Could you check a few things on this model? Use its own coordinates, in mm. Face numbers are marked on the shaded views. A direction names the side the tool comes from. Round coordinates to 2 decimals unless told otherwise and drop trailing zeros. Write each loop counter-clockwise with the first axis right and the second up, starting at its lowest first coordinate (ties: lowest second). Pieces come first, ordered by that corner, then holes. Notation, with made-up numbers: (36, 48.25) -> (56, 48.25) arc R22 ccw to (56, 71.25) -> close; hole circle Ø11 at (-4, 15.5). An arc over 180 degrees is marked (long way). Answer in a Markdown table with one row per item.
from build123d import *

# Parameters (mm, degrees)
BOSS_EXTRUDE1_DEPTH = 9


with BuildPart() as part:
    # Sketch1 → Boss-Extrude1 (new, symmetric)
    with BuildSketch(Plane.XY):
        with BuildLine():
            Line((10, 3.992849301), (10, -6.01853916))
            Line((10, -6.01853916), (5, -6.01853916))
            ThreePointArc((5, -6.01853916), (4.292893219, -6.311432379), (4, -7.01853916))
            Line((4, -7.01853916), (4, -8.007150699))
            Line((4, -8.007150699), (-4, -8.007150699))
            Line((-4, -8.007150699), (-4, -7.01853916))
            ThreePointArc((-4, -7.01853916), (-4.292893219, -6.311432379), (-5, -6.01853916))
            Line((-5, -6.01853916), (-10, -6.01853916))
            Line((-10, -6.01853916), (-10, 3.992849301))
            ThreePointArc((-10, 3.992849301), (0, 1.100511346), (10, 3.992849301))
        make_face()
    extrude(amount=BOSS_EXTRUDE1_DEPTH, both=True)


solid = part.part
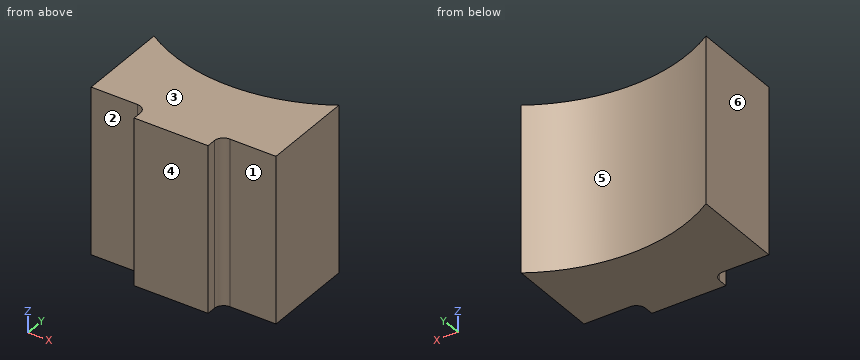
1) Imagine slicing it at A-A, the plane z = 1. Please give me the cut outline in (x, y).
Findings:
| item | result |
|---|---|
| outline | (-10, -6.02) -> (-5, -6.02) arc R1 cw to (-4, -7.02) -> (-4, -8.01) -> (4, -8.01) -> (4, -7.02) arc R1 cw to (5, -6.02) -> (10, -6.02) -> (10, 3.99) arc R18.73 cw to (-10, 3.99) -> close |
2) Thinking about a two-plate mould opening in X: for the marked faces 4, 5 and 6, which applies, +X half, -X half, draft (parallel to the pull), parting line (faces both ways), or undercut?
Findings:
| item | result |
|---|---|
| face 4 | draft |
| face 5 | undercut |
| face 6 | -X half |
3) Please list where these lines run through material, in increasing order: line 1 (X direction, y = 3, z = 2.25); line 2 (Y direction, x = 4.5, z = 2); line 3 (Y direction, x = -2.25, z = -7).
Findings:
| item | result |
|---|---|
| line 1 | x = -10 to -8.22, 8.22 to 10 |
| line 2 | y = -6.15 to 1.65 |
| line 3 | y = -8.01 to 1.24 |
4) Imagine slicing it at B-B, the plane x = 5.25. Please give me the cut outline in (y, z), plus the area to 3 significant figures.
Findings:
| item | result |
|---|---|
| outline | (-6.02, -9) -> (1.85, -9) -> (1.85, 9) -> (-6.02, 9) -> close |
| area | 142 mm^2 |
5) For the marked faces 1, 2 and 3, which set-ups out of +Z, -Z, +X, -X, +Y, -Y let a thin tool reach every point of the face, with its end or its side?
Findings:
| item | result |
|---|---|
| face 1 | +Z, -Z, +X, -Y |
| face 2 | +Z, -Z, -X, -Y |
| face 3 | +Z, +X, -X, +Y, -Y |
6) Imagine slicing it at C-C, the plane x = -8.5. Please give me the cut outline in (y, z), plus the area to 3 significant figures.
Findings:
| item | result |
|---|---|
| outline | (-6.02, -9) -> (3.14, -9) -> (3.14, 9) -> (-6.02, 9) -> close |
| area | 165 mm^2 |
7) For pin 1 (1 mm diameter, centred on x = -3.5, z = 7, fed in from +Y); pin 2 (1.1 mm diameter, centred on y = -7.5, z = -0.5, fed in from -X); pin 3 (4 mm diameter, centred on x = -1.5, z = -2.5, fed in from +Y), each with a flat end and sliding along its axis, tell me the tip position at first contact or that it passes through.
Findings:
| item | result |
|---|---|
| pin 1 | stops at y = 1.53 |
| pin 2 | stops at x = -4 |
| pin 3 | stops at y = 1.43 |
